from build123d import *

# Parameters (mm, degrees)
SKETCH1_W           = 49.2
SKETCH1_H           = 49.2
SKETCH1_W_2         = 42.4
SKETCH1_H_2         = 42.4
BOSS_EXTRUDE1_DEPTH = 10
CHAMFER1_SIZE       = 3.5
FILLET1_R           = 10
CUT_EXTRUDE1_REACH  = 42.129
SKETCH2_W           = 18.6
SKETCH2_H           = 6.8
SKETCH4_W           = 6.8
SKETCH4_H           = 20
BOSS_EXTRUDE2_DEPTH = 20
SKETCH5_R           = 1.6
CUT_EXTRUDE2_DEPTH  = 55.283054446
BOSS_EXTRUDE3_DEPTH = 25
SKETCH8_W           = 39
SKETCH8_H           = 10
BOSS_EXTRUDE4_DEPTH = 10
FILLET3_R           = 10
CUT_EXTRUDE3_REACH  = 100.797
SKETCH10_W          = 19
SKETCH10_H          = 51.482775671
FILLET4_R           = 60
SKETCH11_R          = 3.25
CUT_EXTRUDE4_DEPTH  = 95.979997894
SKETCH15_R          = 4.5
CUT_EXTRUDE6_DEPTH  = 31.25
SKETCH16_R          = 4.5
CUT_EXTRUDE7_DEPTH  = 31.25
BOSS_EXTRUDE5_START = 19.38
SKETCH17_R          = 3.25
BOSS_EXTRUDE5_DEPTH = 19.38
SKETCH18_R          = 4.5
CUT_EXTRUDE8_DEPTH  = 19.38
BOSS_EXTRUDE6_DEPTH = 20
FILLET6_R           = 5
BOSS_EXTRUDE7_DEPTH = 42
FILLET7_R           = 5


with BuildPart() as part:
    # Sketch1 → Boss-Extrude1 (new, symmetric)
    with BuildSketch(Plane.XY):
        Rectangle(SKETCH1_W, SKETCH1_H)
        Rectangle(SKETCH1_W_2, SKETCH1_H_2, mode=Mode.SUBTRACT)
    extrude(amount=BOSS_EXTRUDE1_DEPTH, both=True)

    # Chamfer1
    chamfer1_edges = [part.edges().sort_by_distance(p)[0] for p in [
        (21.2, -21.2, 0),
        (21.2, 21.2, 0),
        (-21.2, 21.2, 0),
        (-21.2, -21.2, 0),
    ]]
    chamfer(chamfer1_edges, length=CHAMFER1_SIZE)

    # Fillet1
    fillet1_edges = [part.edges().sort_by_distance(p)[0] for p in [
        (24.6, -24.6, 0),
        (-24.6, -24.6, 0),
        (-24.6, 24.6, 0),
        (24.6, 24.6, 0),
    ]]
    fillet(fillet1_edges, radius=FILLET1_R)

    # Sketch2 → Cut-Extrude1 (cut, up to next)
    with BuildSketch(Plane.XY.offset(10), mode=Mode.PRIVATE) as cut_extrude1_sk1:
        with Locations((0, 21.2)):
            Rectangle(SKETCH2_W, SKETCH2_H)
    cut_extrude1_tool1 = extrude(cut_extrude1_sk1.sketch, amount=-CUT_EXTRUDE1_REACH, mode=Mode.PRIVATE) & part.part
    add(cut_extrude1_tool1.solids().sort_by_distance((0, 21.2, 10))[0], mode=Mode.SUBTRACT)

    # Sketch4 → Boss-Extrude2 (add)
    with BuildSketch(Plane.XZ.offset(-21.2)):
        with Locations((-5.9, 0)):
            Rectangle(SKETCH4_W, SKETCH4_H)
        with Locations((5.9, 0)):
            Rectangle(SKETCH4_W, SKETCH4_H)
    extrude(amount=-BOSS_EXTRUDE2_DEPTH)

    # Sketch5 → Cut-Extrude2 (cut, through all)
    with BuildSketch(Plane(origin=(9.3, 0, 0), x_dir=(0, 0, -1), z_dir=(1, 0, 0))):
        with Locations((0, 32.9)):
            Circle(SKETCH5_R)
    extrude(amount=-CUT_EXTRUDE2_DEPTH, mode=Mode.SUBTRACT)

    # Sketch7 → Boss-Extrude3 (add)
    with BuildSketch(Plane.XY):
        Polygon((-19.5, -24.6), (-19.5, -84.8), (19.5, -84.8), (19.5, -24.6), (19.5, -23.273751878), (-19.5, -23.317224329), align=None)
    extrude(amount=BOSS_EXTRUDE3_DEPTH)

    # Sketch8 → Boss-Extrude4 (add)
    with BuildSketch(Plane(origin=(0, 0, 0), x_dir=(-1, 0, 0), z_dir=(0, 0, -1))):
        with Locations((0, -28.317224329)):
            Rectangle(SKETCH8_W, SKETCH8_H)
    extrude(amount=BOSS_EXTRUDE4_DEPTH)

    # Fillet3
    fillet3_edges = [part.edges().sort_by_distance(p)[0] for p in [
        (0, -23.295488103, 25),
    ]]
    fillet(fillet3_edges, radius=FILLET3_R)

    # Sketch10 → Cut-Extrude3 (cut, up to next)
    with BuildSketch(Plane.ZY.offset(19.5), mode=Mode.PRIVATE) as cut_extrude3_sk1:
        with Locations((9.5, -59.058612165)):
            Rectangle(SKETCH10_W, SKETCH10_H)
    cut_extrude3_tool1 = extrude(cut_extrude3_sk1.sketch, amount=-CUT_EXTRUDE3_REACH, mode=Mode.PRIVATE) & part.part
    add(cut_extrude3_tool1.solids().sort_by_distance((-19.5, -59.058612, 9.5))[0], mode=Mode.SUBTRACT)

    # Fillet4
    # the kernel refuses this fillet: 60 mm, written as the material it adds along each edge
    with BuildSketch(Plane(origin=(-19.5, -33.317224329, 19), x_dir=(0, -1, 0), z_dir=(1, 0, 0))) as fillet4_piece_1:
        with BuildLine():
            CenterArc((51.371198156, 60), FILLET4_R, 211.108922511, 58.891077489)
            Line((0, 29), (0, 0))
            Line((0, 0), (51.371198156, 0))
        make_face()
    extrude(amount=39)

    # Sketch11 → Cut-Extrude4 (cut, through all)
    with BuildSketch(Plane.XY.offset(25)):
        with Locations((-12.5, -39.8)):
            Circle(SKETCH11_R)
        with Locations((12.5, -39.8)):
            Circle(SKETCH11_R)
        with Locations((-12.5, -78.8)):
            Circle(SKETCH11_R)
        with Locations((12.5, -78.8)):
            Circle(SKETCH11_R)
    extrude(amount=-CUT_EXTRUDE4_DEPTH, mode=Mode.SUBTRACT)

    # Sketch15 → Cut-Extrude6 (cut)
    with BuildSketch(Plane(origin=(0, 0, -10), x_dir=(-1, 0, 0), z_dir=(0, 0, -1))):
        with Locations((-12.5, -39.8)):
            Circle(SKETCH15_R)
        with Locations((12.5, -39.8)):
            Circle(SKETCH15_R)
    extrude(amount=-CUT_EXTRUDE6_DEPTH, mode=Mode.SUBTRACT)

    # Sketch16 → Cut-Extrude7 (cut)
    with BuildSketch(Plane(origin=(0, 0, -10), x_dir=(-1, 0, 0), z_dir=(0, 0, -1))):
        with Locations((-12.5, -78.8)):
            Circle(SKETCH16_R)
        with Locations((12.5, -78.8)):
            Circle(SKETCH16_R)
    extrude(amount=-CUT_EXTRUDE7_DEPTH, mode=Mode.SUBTRACT)

    # Sketch17 → Boss-Extrude5 (add)
    with BuildSketch(Plane.XY.offset(25).offset(BOSS_EXTRUDE5_START)):
        Polygon((19.5, -84.8), (19.5, -33.27375809), (-19.5, -33.317230541), (-19.5, -84.8), align=None)
        with Locations((-12.5, -78.8)):
            Circle(SKETCH17_R, mode=Mode.SUBTRACT)
        with Locations((12.5, -78.8)):
            Circle(SKETCH17_R, mode=Mode.SUBTRACT)
        with Locations((12.5, -39.8)):
            Circle(SKETCH17_R, mode=Mode.SUBTRACT)
        with Locations((-12.5, -39.8)):
            Circle(SKETCH17_R, mode=Mode.SUBTRACT)
    extrude(amount=-BOSS_EXTRUDE5_DEPTH)

    # Sketch18 → Cut-Extrude8 (cut)
    with BuildSketch(Plane(origin=(0, 0, 21.25), x_dir=(-1, 0, 0), z_dir=(0, 0, -1))):
        with Locations((12.5, -78.8)):
            Circle(SKETCH18_R)
        with Locations((-12.5, -78.8)):
            Circle(SKETCH18_R)
        with Locations((12.5, -39.8)):
            Circle(SKETCH18_R)
        with Locations((-12.5, -39.8)):
            Circle(SKETCH18_R)
    extrude(amount=-CUT_EXTRUDE8_DEPTH, mode=Mode.SUBTRACT)

    # Sketch20 → Boss-Extrude6 (add)
    with BuildSketch(Plane.XY.offset(10)):
        with BuildLine():
            Line((64.6, 24.6), (14.6, 24.6))
            ThreePointArc((14.6, 24.6), (21.671067812, 21.671067812), (24.6, 14.6))
            Line((24.6, 14.6), (24.6, -14.6))
            ThreePointArc((24.6, -14.6), (23.253481333, -19.611712364), (19.576547836, -23.273751878))
            Line((19.576547836, -23.273751878), (64.6, -23.273751878))
            Line((64.6, -23.273751878), (64.6, 24.6))
        make_face()
    extrude(amount=-BOSS_EXTRUDE6_DEPTH)

    # Fillet6
    fillet6_edges = [part.edges().sort_by_distance(p)[0] for p in [
        (64.6, -23.273751878, 0),
        (64.6, 24.6, 0),
    ]]
    fillet(fillet6_edges, radius=FILLET6_R)

    # Sketch21 → Boss-Extrude7 (add)
    with BuildSketch(Plane.XY.offset(10)):
        with BuildLine():
            Line((24.6, 24.6), (24.6, -23.273751878))
            Line((24.6, -23.273751878), (59.6, -23.273751878))
            ThreePointArc((59.6, -23.273751878), (63.135533906, -21.809285784), (64.6, -18.273751878))
            Line((64.6, -18.273751878), (64.6, 19.6))
            ThreePointArc((64.6, 19.6), (63.135533906, 23.135533906), (59.6, 24.6))
            Line((59.6, 24.6), (24.6, 24.6))
        make_face()
    extrude(amount=BOSS_EXTRUDE7_DEPTH)

    # Fillet7
    fillet7_edges = [part.edges().sort_by_distance(p)[0] for p in [
        (24.6, 24.6, 31),
        (24.6, -23.273751878, 31),
    ]]
    fillet(fillet7_edges, radius=FILLET7_R)


with BuildPart() as body_2:
    # Mirror1: mirrored copy
    add(part.part.mirror(Plane(origin=(-24.6, -24.6, 10), x_dir=(0, 0, 1), z_dir=(1, 0, 0))))


solid = body_2.part
Can you work these out from the model? Positions are in its coordinate system, mm. A direction names the side the tool comes from. Give positions to 0.01 mm unless a question says otherwise; leave off trailing zeros. Order: outer loops, then holes, each group sorted by start corner. A loop starts at its lowest first (then second) coordinate and runs counter-clockwise, first axis right, second up. Notation, with made-up numbers: M 71.25,38.25 L 80.25,38.25 A23 cw 80.25,53.25 Z; hole C -13,-17.75 d6. An arc over 180 degrees is marked long. Use a Markdown table: item, result. Add a question column.
Item 1: We'd pull the mould along Y, two halves only. Please class faces 5 (the cylindrical face through (-35.995, -81.973, 42.531)), 6 (the flat face through (-68.6, -19.5, 0.1)), 7 (the flat face through (-43, 41.2, 0)), 8 (the flat face through (-51.7, 31, 0)): +Y half, -Y half, draft (parallel to the pull), parting line (faces both ways), or undercut.
Item 2: Suppose I cut it at B-B (y = 32.9). List the corners of the cut face in (x, z) for me.
Item 3: Suppose I cut it at C-C (y = -39.8). List the corners of the cut face in (x, z) for me, then the cut area to 3 significant figures.
Item 4: If I drill on L1, parallel to Y at x = -36.7, z = 26.5; L2, parallel to X at y = -78.8, z = 35.75; L3, parallel to Y at x = -54, z = 0, over which ranges is the centre line in solid material (lowest first)? Write a range as [from, to].
Item 5: Suppose I cut it at A-A (z = 28.5). List the corners of the cut face in (x, y) for me.
Item 6: Will these pins go through, and if not, where does the flat tip stop? pin 1 (7.5 mm diameter, centred on x = -36.7, y = -78.8, fed in from -Z); pin 2 (10 mm diameter, centred on y = 32, z = 3, fed in from -X); pin 3 (10 mm diameter, centred on y = -25.5, z = 44.5, fed in from +X).
Item 7: Suppose I cut it at D-D (x = -43.5). Count the separate pieces of the cut face and the enclosed holes in it, then the cut area to 3 significant figures.
Item 8: For faces 1 (the cylindrical face through (-75.23, 23.1, 31.29)), 2 (the flat face through (-70.4, 0, 0)), 3 (the flat face through (-29.7, -54, 24)), 4 (the flat face through (-93, -23.274, 21)), which set-ups out of +Z, -Z, +X, -X, +Y, -Y let a thin tool reach every point of the face, with its end or its side?
Answer sheet:
| question | item | result |
|---|---|---|
| 1 | face 5 | undercut |
| 1 | face 6 | undercut |
| 1 | face 7 | +Y half |
| 1 | face 8 | draft |
| 2 | outline | M -58.5,-10 L -51.7,-10 L -51.7,-1.6 L -58.5,-1.6 Z; M -58.5,1.6 L -51.7,1.6 L -51.7,10 L -58.5,10 Z; M -46.7,-10 L -39.9,-10 L -39.9,-1.6 L -46.7,-1.6 Z; M -46.7,1.6 L -39.9,1.6 L -39.9,10 L -46.7,10 Z |
| 3 | outline | M -68.7,-1.19 L -66.2,-1.19 L -66.2,40.63 L -64.95,40.63 L -64.95,44.38 L -68.7,44.38 Z; M -58.45,40.63 L -57.2,40.63 L -57.2,-1.19 L -41.2,-1.19 L -41.2,40.63 L -39.95,40.63 L -39.95,44.38 L -58.45,44.38 Z; M -33.45,40.63 L -32.2,40.63 L -32.2,-1.19 L -29.7,-1.19 L -29.7,44.38 L -33.45,44.38 Z |
| 3 | area | 976 mm² |
| 4 | L1 | y = [-84.8, -83.3], [-74.3, -44.3], [-35.3, -33.31] |
| 4 | L2 | x = [-68.7, -66.2], [-57.2, -41.2], [-32.2, -29.7] |
| 4 | L3 | y = [-40.88, -21.2], [21.2, 31.3], [34.5, 41.2] |
| 5 | outline | M -113.8,-18.27 A5 ccw -108.8,-23.27 L -78.8,-23.27 A5 ccw -73.8,-18.27 L -73.8,19.6 A5 ccw -78.8,24.6 L -108.8,24.6 A5 ccw -113.8,19.6 Z; M -68.7,-84.8 L -29.7,-84.8 L -29.7,-33.32 L -68.7,-33.27 Z; hole C -61.7,-78.8 d9; hole C -61.7,-39.8 d9; hole C -36.7,-78.8 d9; hole C -36.7,-39.8 d9 |
| 6 | pin 1 | stops at z = 40.63 |
| 6 | pin 2 | stops at x = -58.5 |
| 6 | pin 3 | stops at x = -74.32 |
| 7 | separate pieces | 2 |
| 7 | enclosed holes | 1 |
| 7 | area | 2,510 mm² |
| 8 | face 1 | +Z, +X, +Y |
| 8 | face 2 | +Z, -Z |
| 8 | face 3 | +Z, -Z, +X, -Y |
| 8 | face 4 | +Z, -Z, -X, -Y |
